Check sheet for the modelled part. Datum: model origin and axes. Units: mm. A direction names the side the tool comes from. Coordinates: 2 decimals unless noted, no trailing zeros. Loops run counter-clockwise (first coordinate to the right, second up) from the corner with the lowest first, then second, coordinate; pieces in that order, holes last. Notation, with made-up numbers: M 53,76 L 60,76 A17 ccw 60,105 Z; hole C 58.5,33 d10. An arc over 180 degrees is marked long. Use CSV: the item, a comma, the result in double quotes. Start each with the question number.
(1) Section check C-C on y = 34.29. Record the cut outline in (x, z).
(2) Section check A-A on y = 8. Record the cut outline in (x, z).
(3) Go/stop test with flat-tipped pins: pin 1 Ø0.8 at (y, z) = (34, 13) entering from +X; pin 2 Ø5 at (x, z) = (1.5, 18.5) entering from +Y; pin 3 Ø3 at (y, z) = (32.5, 9.5) entering from +X; pin 4 Ø1 at (x, y) = (7, 24) entering from -Z. Record where each tip stops, or that it passes through.
(4) Section check D-D on x = 4.5. Record the cut outline in (y, z).
(5) Section check B-B on z = 18.25. Give the number of separate pieces and of enclosed holes in the cut face, and give its area (3 significant figures).
(6) Scan lines: line 1 (X direction, y = 7, z = 8.75); line 2 (Y direction, x = 24.5, z = 2); line 3 (X direction, y = 35, z = 9.25). Record each from-to range of solid material in increasing order.
(7) Draft check along Y on faces 1 (the flat face through (13, -10.16, 13)), 2 (the cylindrical face through (7.584, 34.262, 3.493)), 3 (the cylindrical face through (21.044, 31.244, 12.522)), 4 (the flat face through (20.32, 34, 13)). Enter one of: pulls with the +Y half, pulls with the -Y half, needs draft (parallel to the pull), parting line crosses it, or undercut.
(8) Set-up check for faces 5 (the cylindrical face through (15.964, 26.164, 12.522)), 6 (the flat face through (20.32, 34, 24)), 7 (the flat face through (15.24, 33, 13)): record each of +Z, -Z, +X, -X, +Y, -Y from which the full face is reachable in a straight line by a thin tool's end or side.
from build123d import *

# Parameters (mm, degrees)
SKETCH1_W                = 25.4
SKETCH1_H                = 25.4
BOSS_EXTRUDE1_DEPTH      = 25.4
SKETCH2_W                = 5.08
SKETCH2_H                = 5.08
CUT_EXTRUDE1_DEPTH       = 51.032197633
FILLET1_R                = 2.54
SKETCH3_W                = 5.08
SKETCH3_H                = 7.62
BOSS_EXTRUDE2_DEPTH      = 25.4
FILLET2_R                = 2.54
CUT_EXTRUDE2_DEPTH       = 53.363441445
BOSS_EXTRUDE3_DEPTH      = 5.08
BOSS_EXTRUDE3_DEPTH_BACK = 5.08
SKETCH5_W                = 35.56
SKETCH5_H                = 25.4
FILLET3_R                = 5.08


with BuildPart() as part:
    # Sketch1 → Boss-Extrude1 (new body)
    with BuildSketch(Plane.XY):
        with BuildLine():
            Line((-5.08, 0), (-5.08, 25.4))
            ThreePointArc((-5.08, 25.4), (-3.592102448, 28.992102448), (0, 30.48))
            Line((0, 30.48), (25.4, 30.48))
            ThreePointArc((25.4, 30.48), (28.992102448, 28.992102448), (30.48, 25.4))
            Line((30.48, 25.4), (30.48, 0))
            ThreePointArc((30.48, 0), (28.992102448, -3.592102448), (25.4, -5.08))
            Line((25.4, -5.08), (0, -5.08))
            ThreePointArc((0, -5.08), (-3.592102448, -3.592102448), (-5.08, 0))
        make_face()
        with Locations((12.7, 12.7)):
            Rectangle(SKETCH1_W, SKETCH1_H, mode=Mode.SUBTRACT)
    extrude(amount=BOSS_EXTRUDE1_DEPTH)

    # Sketch2 → Cut-Extrude1 (cut, through all)
    with BuildSketch(Plane.XY.offset(25.4)):
        with Locations((12.7, 27.94)):
            Rectangle(SKETCH2_W, SKETCH2_H)
    extrude(amount=-CUT_EXTRUDE1_DEPTH, mode=Mode.SUBTRACT)

    # Fillet1
    fillet1_edges = [part.edges().sort_by_distance(p)[0] for p in [
        (10.16, 25.4, 12.7),
        (15.24, 25.4, 12.7),
    ]]
    fillet(fillet1_edges, radius=FILLET1_R)

    # Sketch3 → Boss-Extrude2 (add)
    with BuildSketch(Plane.XY.offset(25.4)):
        with Locations((7.62, 34.29)):
            Rectangle(SKETCH3_W, SKETCH3_H)
        with Locations((17.78, 34.29)):
            Rectangle(SKETCH3_W, SKETCH3_H)
    extrude(amount=-BOSS_EXTRUDE2_DEPTH)

    # Fillet2
    fillet2_edges = [part.edges().sort_by_distance(p)[0] for p in [
        (5.08, 30.48, 12.7),
        (5.08, 38.1, 12.7),
        (20.32, 38.1, 12.7),
        (20.32, 30.48, 12.7),
    ]]
    fillet(fillet2_edges, radius=FILLET2_R)

    # Sketch4 → Cut-Extrude2 (cut, through all)
    with BuildSketch(Plane.ZY.offset(-5.08)):
        with BuildLine():
            Line((4.7625, 35.56), (7.9375, 35.56))
            ThreePointArc((7.9375, 35.56), (9.2075, 34.29), (7.9375, 33.02))
            Line((7.9375, 33.02), (4.7625, 33.02))
            ThreePointArc((4.7625, 33.02), (3.4925, 34.29), (4.7625, 35.56))
        make_face()
        with BuildLine():
            Line((17.4625, 35.56), (20.6375, 35.56))
            ThreePointArc((20.6375, 35.56), (21.9075, 34.29), (20.6375, 33.02))
            Line((20.6375, 33.02), (17.4625, 33.02))
            ThreePointArc((17.4625, 33.02), (16.1925, 34.29), (17.4625, 35.56))
        make_face()
    extrude(amount=-CUT_EXTRUDE2_DEPTH, mode=Mode.SUBTRACT)

    # Sketch5 → Boss-Extrude3 (add, two sides: drawn at the far end of the back side and taken through both)
    with BuildSketch(Plane.XZ.offset(5.08).offset(-BOSS_EXTRUDE3_DEPTH_BACK)):
        with Locations((12.7, 12.7)):
            Rectangle(SKETCH5_W, SKETCH5_H)
    extrude(amount=BOSS_EXTRUDE3_DEPTH + BOSS_EXTRUDE3_DEPTH_BACK)

    # Fillet3
    fillet3_edges = [part.edges().sort_by_distance(p)[0] for p in [
        (-5.08, -10.16, 12.7),
        (30.48, -10.16, 12.7),
    ]]
    fillet(fillet3_edges, radius=FILLET3_R)


solid = part.part
Outcome:
1,outline,"M 5.08,0 L 10.16,0 L 10.16,3.49 L 5.08,3.49 Z; M 5.08,9.21 L 10.16,9.21 L 10.16,16.19 L 5.08,16.19 Z; M 5.08,21.91 L 10.16,21.91 L 10.16,25.4 L 5.08,25.4 Z; M 15.24,0 L 20.32,0 L 20.32,3.49 L 15.24,3.49 Z; M 15.24,9.21 L 20.32,9.21 L 20.32,16.19 L 15.24,16.19 Z; M 15.24,21.91 L 20.32,21.91 L 20.32,25.4 L 15.24,25.4 Z"
2,outline,"M -5.08,0 L 0,0 L 0,25.4 L -5.08,25.4 Z; M 25.4,0 L 30.48,0 L 30.48,25.4 L 25.4,25.4 Z"
3,pin 1,"stops at x = 20.32"
3,pin 2,"stops at y = 30.94"
3,pin 3,"stops at x = 21.32"
3,pin 4,"passes through"
4,outline,"M -10.16,0 L 0,0 L 0,25.4 L -10.16,25.4 Z; M 25.4,0 L 31.4,0 L 31.4,25.4 L 25.4,25.4 Z"
5,separate pieces,"3"
5,enclosed holes,"0"
5,area,"801 mm²"
6,line 1,"x = -5.08 to 0, 25.4 to 30.48"
6,line 2,"y = -10.16 to 0, 25.4 to 30.48"
6,line 3,"x = 5.08 to 10.16, 15.24 to 20.32"
7,face 1,"pulls with the -Y half"
7,face 2,"undercut"
7,face 3,"pulls with the +Y half"
7,face 4,"needs draft"
8,face 5,"+Z, -Z"
8,face 6,"+Z, -Z, +X, +Y"
8,face 7,"+Z, -Z, +Y"
